Autodesk Inventor part; units mm, degrees
ref_plane "YZ Plane" through (0, 0, 0) normal (1, 0, 0) x (0, 1, 0)
ref_plane "XZ Plane" through (0, 0, 0) normal (0, 1, 0) x (-1, 0, 0)
ref_plane "XY Plane" through (0, 0, 0) normal (0, 0, 1) x (1, 0, 0)
ref_plane "Plano de trabajo1" through (0, 0, 0) normal (0, 0, 1) x (1, 0, 0)
sketch "Boceto1" plane through (0, 0, 0) normal (0, 0, 1) x (1, 0, 0)
  circle A0 centre (10.9923, 0) radius 10.9823
  circle A1 centre (10.9923, 7.35) radius 1.2028
  circle A2 centre (3.6423, 0) radius 1.2028
  circle A3 centre (18.3423, 0) radius 1.2028
  circle A4 centre (18.7153, -9.5116) radius 1.05
  circle A5 centre (10.9923, -7.35) radius 1.2028
  line L0 (10.9923, 0) -> (160.9923, 0)
  line L1 (10.9923, 10.9823) -> (160.9923, 10.9823)
  line L2 (10.9923, -10.9823) -> (160.9923, -10.9823)
  line L3 (160.9923, -10.9823) -> (160.9923, 10.9823)
  point P0 (0, 0)
  dimension "d0" = 150
extrude "Extrusión1" add sketch "Boceto1" along normal blind 3
sketch "Boceto2" plane through (0, 0, 3) normal (0, 0, 1) x (1, 0, 0)
  arc A0 (151.1597, 5.5871) -> (154.1073, 8.4343) centre (150.0864, 9.6477) ccw
  circle A1 centre (150.0864, -8.5523) radius 0.85
  circle A2 centre (150.0864, 9.6477) radius 0.85
  line L0 (160.9923, 10.9823) -> (10.9923, 10.9823)
  line L1 (10.9923, -10.9823) -> (160.9923, -10.9823)
  line L2 (160.9923, -10.9823) -> (160.9923, 10.9823)
  line L3 (160.9923, 10.9823) -> (10.9923, 10.9823)
  arc A3 (10.9923, 10.9823) -> (10.9923, -10.9823) centre (10.9923, 0) ccw
  circle A4 centre (18.7153, -9.5116) radius 1.05
  circle A5 centre (10.9923, 7.35) radius 1.2028
  circle A6 centre (3.6423, 0) radius 1.2028
  circle A7 centre (10.9923, -7.35) radius 1.2028
  circle A8 centre (18.3423, 0) radius 1.2028
  line L4 (150.0864, 10.9823) -> (150.0864, -0.0002)
  line L5 (150.0864, -0.0002) -> (150.0864, -9.1002)
  line L6 (150.0864, -0.0002) -> (150.0864, 9.0998)
  circle A9 centre (150.0864, 9.0998) radius 0.85
  circle A10 centre (150.0864, -9.1002) radius 0.85
  circle A11 centre (150.0864, 9.0998) radius 1.8825
  circle A12 centre (150.0864, -9.1002) radius 1.8821
  point P0 (0, 0)
  point P1 (150.0864, 7.2173)
  point P2 (150.0864, -7.218)
  point P3 (150.0864, -10.9823)
  dimension "d3" = 10.9825
  dimension "d4" = 9.1
  dimension "d5" = 9.1
  dimension "d6" = 1.7
  dimension "d7" = 1.7
extrude "Extrusión2" cut sketch "Boceto2" against normal blind 3 contours A10 A1 | A1 A10 | A9 L4 A2 | A2 L4 A9 | A9 L4 A2 | A2 L4 A9 | L0 L2 L1 A12 L5 L4 A11 picked at (150.2191, 8.6309) picked at (150.5614, 9.2824) picked at (149.6114, 9.2824) picked at (149.9501, 8.6317)
sketch "Boceto3" plane through (0, 0, 3) normal (0, 0, 1) x (1, 0, 0)
  point P0 (0, 0)
sketch "Boceto4" plane through (0, 0, 3) normal (0, 0, 1) x (1, 0, 0)
  circle A0 centre (18.7153, -9.5116) radius 1.05
  point P0 (0, 0)
extrude "Extrusión3" add sketch "Boceto4" against normal blind 3
sketch "Boceto5" plane through (0, 0, 3) normal (0, 0, 1) x (1, 0, 0)
  circle A0 centre (150.0864, 9.0998) radius 0.85
  circle A1 centre (150.0864, -9.1002) radius 0.85
  circle A2 centre (150.0864, 9.0998) radius 2.6325
  circle A3 centre (150.0864, -9.1002) radius 2.632
  line L0 (150.0864, -7.218) -> (150.0864, 7.2173)
  circle A4 centre (18.3423, 0) radius 1.2028
  circle A5 centre (10.9923, -7.35) radius 1.2028
  circle A6 centre (3.6423, 0) radius 1.2028
  circle A7 centre (10.9923, 7.35) radius 1.2028
  arc A8 (150.0864, -10.9823) -> (150.0864, -7.218) centre (150.0864, -9.1002) ccw
  line L1 (150.0864, -7.218) -> (150.0864, 7.2173)
  arc A9 (150.0864, 7.2173) -> (150.0864, 10.9823) centre (150.0864, 9.0998) ccw
  line L2 (150.0864, 10.9823) -> (10.9923, 10.9823)
  arc A10 (10.9923, 10.9823) -> (10.9923, -10.9823) centre (10.9923, 0) ccw
  line L3 (10.9923, -10.9823) -> (150.0864, -10.9823)
  circle A11 centre (150.0864, -9.1002) radius 0.85
  circle A12 centre (150.0864, 9.0998) radius 0.85
  point P0 (0, 0)
  point P1 (148.2466, -10.9823)
  point P2 (150.0864, -6.4682)
  point P3 (150.0864, 6.4673)
  point P4 (148.2462, 10.9823)
  dimension "d12" = 5.265
  dimension "d13" = 5.264
extrude "Extrusión4" add sketch "Boceto5" against normal blind 3 contours A2 L0 A9 L2 | A3 L3 A8 L0 picked at (149.0222, 11.1076) picked at (149.0224, -11.1076)
properties part number "tibiaMot"
CAD build for the part. Positions are in the model's coordinates, mm. A direction names the side the tool comes from. Round coordinates to 2 decimals unless told otherwise and drop trailing zeros. Order: outer loops, then holes, each group sorted by start corner. A loop starts at its lowest first (then second) coordinate and runs counter-clockwise, first axis right, second up.
Q1. Slice it at B-B (x = 31.5). Write the cut outline in (y, z), and give its area (3 significant figures).
Q2. Slice it at A-A (z = 1.45). State how many separate pieces and enclosed holes the cut face has, and give its area (3 significant figures).
Q3. Two-plate mould, pull along X, no slides. Class faces 1 (the cylindrical face through (2.44, -0.05, 1.48)), 2 (the cylindrical face through (152.55, 10.03, 1.52)), 3 (the cylindrical face through (0.013, -0.241, 1.479)), 4 (the flat face through (79, 10.982, 1)): pulls with the +X half, pulls with the -X half, needs draft (parallel to the pull), parting line crosses it, or undercut.
Q4. Drop flat-ended pins along their axis: pin 1 (0.9 mm diameter, centred on y = 2.5, z = 1, fed in from +X); pin 2 (1.4 mm diameter, centred on x = 150.09, y = -9.1, fed in from +Z). Give the stop position or say it passes through.
Q5. Which spindle directions (+Z, -Z, +X, -X, +Y, -Y) get a long thin tool onto all of the face, cutting with end or side? Do faces 5 (the flat face through (150.086, 0, 2)), 6 (the cylindrical face through (152.496, -10.16, 1.521)), 7 (the flat face through (79, -10.982, 1)). Say none if no direction does.
Q6. Wall check: L1, parallel to Y at x = 11, z = 1.45; L2, parallel to Y at x = 146, z = 1.95; L3, parallel to X at y = -5, z = 0.75. Give the ranges that are in metal, low to high.
Results below:
1. outline: (-10.98, 0) - (10.98, 0) - (10.98, 3) - (-10.98, 3) - close
1. area: 65.9 mm2
2. separate pieces: 1
2. enclosed holes: 6
2. area: 3,250 mm2
3. face 1: undercut
3. face 2: parting line crosses it
3. face 3: pulls with the -X half
3. face 4: needs draft
4. pin 1: stops at x = 150.09
4. pin 2: passes through
5. face 5: +Z, -Z, +X
5. face 6: +Z, -Z
5. face 7: +Z, -Z, -X, -Y
6. L1: y = -10.98 to -8.55, -6.15 to 6.15, 8.55 to 10.98
6. L2: y = -10.98 to 10.98
6. L3: x = 1.21 to 150.09
